from build123d import *

# Parameters (mm, degrees)
SKETCH_2_W               = 228
SKETCH_2_H               = 88
EXTRUDE_1_DEPTH          = 40
SKETCH_3_W               = 92
SKETCH_3_H               = 88
EXTRUDE_2_DEPTH          = 40
CUT_EXTRUDE_1_REACH      = 259.154
SKETCH_4_R               = 31.5
HOLE_WIZARD_M8_3_D       = 6.8
HOLE_WIZARD_M8_3_DEPTH   = 30
HOLE_WIZARD_M8_3_TIP     = 2.042926105
CUT_EXTRUDE_3_REACH      = 259.154
CUT_EXTRUDE_3_END_RADIUS = 31.5
SKETCH_8_R               = 4


with BuildPart() as part:
    # 草图2 → 凸台-拉伸1 (new body)
    with BuildSketch(Plane(origin=(0, 0, 0), x_dir=(1, 0, 0), z_dir=(0, 1, 0))):
        with Locations((114, 44)):
            Rectangle(SKETCH_2_W, SKETCH_2_H)
    extrude(amount=EXTRUDE_1_DEPTH)

    # 草图3 → 凸台-拉伸2 (add)
    with BuildSketch(Plane(origin=(0, 40, 0), x_dir=(1, 0, 0), z_dir=(0, 1, 0))):
        with Locations((46, 44)):
            Rectangle(SKETCH_3_W, SKETCH_3_H)
    extrude(amount=EXTRUDE_2_DEPTH)

    # 草图4 → 切除-拉伸1 (cut, up to next)
    with BuildSketch(Plane(origin=(0, 80, 0), x_dir=(1, 0, 0), z_dir=(0, 1, 0)), mode=Mode.PRIVATE) as cut_extrude_1_sk1:
        with Locations(Location((46.5, 44, 0), (0, 0, 270))):
            Circle(SKETCH_4_R)
    cut_extrude_1_tool1 = extrude(cut_extrude_1_sk1.sketch, amount=-CUT_EXTRUDE_1_REACH, mode=Mode.PRIVATE) & part.part
    add(cut_extrude_1_tool1.solids().sort_by_distance((46.5, 80, -44))[0], mode=Mode.SUBTRACT)

    # M8 螺纹孔3
    with Locations(Plane(origin=(0, 80, 0), x_dir=(1, 0, 0), z_dir=(0, 1, 0))):
        with Locations((74.077164466, 71.577164466), (8.828892775, 54.093942759), (18.922835534, 16.422835534), (8.828892775, 33.906057241), (74.077164466, 16.422835534), (18.922835534, 71.577164466), (84.171107225, 33.906057241), (84.171107225, 54.093942759)):
            Hole(HOLE_WIZARD_M8_3_D / 2, depth=HOLE_WIZARD_M8_3_DEPTH)
            with Locations((0, 0, -(HOLE_WIZARD_M8_3_DEPTH + HOLE_WIZARD_M8_3_TIP / 2))):  # 118° drill point
                Cone(0, HOLE_WIZARD_M8_3_D / 2, HOLE_WIZARD_M8_3_TIP, mode=Mode.SUBTRACT)

    # 切除-拉伸3: up to this cylinder (the profile starts outside it)
    cut_extrude_3_end = Plane(origin=(46.5, 55.496491, -44), z_dir=(0, 1, 0)) * Cylinder(CUT_EXTRUDE_3_END_RADIUS, 582.308, mode=Mode.PRIVATE)
    # 草图8 → 切除-拉伸3 (cut, up to the surface)
    with BuildSketch(Plane.XY, mode=Mode.PRIVATE) as cut_extrude_3_sk1:
        with Locations((46, 55.496491008)):
            Circle(SKETCH_8_R)
    cut_extrude_3_tool1 = extrude(cut_extrude_3_sk1.sketch, amount=-CUT_EXTRUDE_3_REACH, mode=Mode.PRIVATE) - cut_extrude_3_end
    add(cut_extrude_3_tool1.solids().sort_by_distance((46, 55.496491, 0))[0], mode=Mode.SUBTRACT)


solid = part.part
Input: part model. Units: mm. Frame: model coordinates. A direction names the side the tool comes from. Give positions to 0.01 mm unless a question says otherwise; leave off trailing zeros. Order: outer loops, then holes, each group sorted by start corner. A loop starts at its lowest first (then second) coordinate and runs counter-clockwise, first axis right, second up. Notation, with made-up numbers: M 65.25,81 L 109.25,81 A17 cw 109.25,102 Z; hole C 37,-6 d7. An arc over 180 degrees is marked long. Answer as a JSON object with one key per item and string values.
1. First-contact query: P1, Ø4, axis at y = 40, z = -35, coming from the -X side; P2, Ø6, axis at x = 74.08, z = -71.58, coming from the +Y side; P3, Ø1, axis at x = 122.5, z = -58.5, coming from the +Y side; P4, Ø5.5, axis at x = 74.08, z = -16.42, coming from the +Y side. Flat tips, straight axial feed; report the tip coordinate or a pass-through.
Result sheet:
{"P1": "x = 0", "P2": "y = 49.76", "P3": "y = 40", "P4": "y = 49.61"}
2. Cut plane D-D, the plane z = -80. Output: boundary loops of the cut face in (x, y), and give its area (3 significant figures).
Result sheet:
{"outline": "M 0,0 L 228,0 L 228,40 L 92,40 L 92,80 L 0,80 Z", "area": "12,800 mm²"}
3. Cut plane C-C, the plane y = 22.5. Output: boundary loops of the cut face in (x, z).
Result sheet:
{"outline": "M 0,-88 L 228,-88 L 228,0 L 0,0 Z; hole C 46.5,-44 d63"}
4. Pull-direction query (X, two-part tool) for faces 4 (the conical face through (18.795, 48.312, -71.001)), 5 (the flat face through (92, 60, -43)), 6 (the flat face through (87, 31, -88)); classes: +X half, -X half, draft (parallel to the pull), parting line (faces both ways), or undercut.
Result sheet:
{"face 4": "undercut", "face 5": "+X half", "face 6": "draft"}
5. Ray query, line 1 (Z direction, x = 41, y = 17.5); line 2 (X direction, y = 67.5, z = -54.5); line 3 (X direction, y = 28, z = -44). Return the intervals inside material, ascending. Write a range as [from, to].
Result sheet:
{"line 1": "[-88, -75.02], [-12.98, 0]", "line 2": "[0, 5.45], [12.2, 16.8], [76.2, 80.8], [87.55, 92]", "line 3": "[0, 15], [78, 228]"}
6. Cut plane B-B, the plane x = 25. Output: boundary loops of the cut face in (y, z).
Result sheet:
{"outline": "M 0,-88 L 80,-88 L 80,-67.02 L 0,-67.02 Z; M 0,-20.98 L 80,-20.98 L 80,0 L 0,0 Z"}
7. Reachability of faces 1 (the flat face through (112, 0, -45)), 2 (the cylindrical face through (70.834, 64.79, -72.598)), 3 (the flat face through (159, 40, -45)) from +Z, -Z, +X, -X, +Y, -Y: full face, straight path, thin tool, end or side. Return the list, or none.
Result sheet:
{"face 1": "+Z, -Z, +X, -X, -Y", "face 2": "+Y", "face 3": "+Z, -Z, +X, +Y"}
8. Cut plane A-A, the plane z = -44. Output: boundary loops of the cut face in (x, y), and give its area (3 significant figures).
Result sheet:
{"outline": "M 0,0 L 15,0 L 15,80 L 0,80 Z; M 78,0 L 228,0 L 228,40 L 92,40 L 92,80 L 78,80 Z", "area": "7,760 mm²"}
